For this review, take the finished solid that the model builds, in its own axes (mm). Coordinates: 2 decimals unless noted, no trailing zeros. Write each loop counter-clockwise with the first axis right and the second up, starting at its lowest first coordinate (ties: lowest second). Pieces come first, ordered by that corner, then holes. Notation, with made-up numbers: (-8, 1.5) -> (19, 1.5) arc R28 ccw to (19, 25.5) -> close; hole circle Ø9 at (-39, -37.75). An arc over 180 degrees is marked (long way). Put each result on its own line as item: value. Start each with the question number.
Item 1: Insertion check: P1, Ø1.5, axis at x = 136, y = -2.5, coming from the +Z side. The pin has a flat end and moves straight along its axis. Give the tip position at first contact, or say it passes through.
Item 2: To check wall thickness, follow L1, parallel to Y at x = -21.75, z = 3.15; L2, parallel to X at y = -105, z = 1.25; L3, parallel to Y at x = 175, z = 1. State the ranges of each line that lie inside material, in increasing order.
Item 3: Consider section A-A on y = -95. Give the boundary of the cut face in (x, z), and give its area (3 significant figures).
Item 4: Consider section B-B on z = 5.1. Give the number of separate pieces and of enclosed holes in the cut face, and give its area (3 significant figures).
```python
from build123d import *

# Parameters (mm, degrees)
ESQUISSE1_W             = 280
ESQUISSE1_H             = 200
EXTRUSION1_DEPTH        = 6
ESQUISSE2_W             = 6.5
ESQUISSE2_H             = 140
ENL_V_MAT_EXTRU_1_DEPTH = 2
ESQUISSE3_R             = 1.6
ENL_V_MAT_EXTRU_2_DEPTH = 2
ENL_V_MAT_EXTRU_4_DEPTH = 2
CONG_1_R                = 2.1
ESQUISSE6_W             = 25
ESQUISSE6_H             = 6.5
ESQUISSE6_W_2           = 75.5
ENL_V_MAT_EXTRU_5_DEPTH = 2
ESQUISSE7_R             = 1.6
ENL_V_MAT_EXTRU_6_DEPTH = 2
ESQUISSE4_R             = 1.05
ENL_V_MAT_EXTRU_3_DEPTH = 273.095571445


with BuildPart() as part:
    # Esquisse1 → Extrusion1 (new body)
    with BuildSketch(Plane.XY):
        with Locations((80, -60)):
            Rectangle(ESQUISSE1_W, ESQUISSE1_H)
    extrude(amount=EXTRUSION1_DEPTH)

    # Esquisse2 → Enlèv. mat.-Extru.1 (cut)
    with BuildSketch(Plane.XY.offset(6)):
        with Locations((-21.75, -60)):
            Rectangle(ESQUISSE2_W, ESQUISSE2_H)
        with Locations((54.75, -60)):
            Rectangle(ESQUISSE2_W, ESQUISSE2_H)
        with Locations((131.25, -60)):
            Rectangle(ESQUISSE2_W, ESQUISSE2_H)
    extrude(amount=-ENL_V_MAT_EXTRU_1_DEPTH, mode=Mode.SUBTRACT)

    # Esquisse3 → Enlèv. mat.-Extru.2 (cut)
    with BuildSketch(Plane.XY.offset(6)):
        with Locations((-23.9, 8.9)):
            Circle(ESQUISSE3_R)
        with Locations((-19.6, 8.9)):
            Circle(ESQUISSE3_R)
        with Locations((-23.9, -128.9)):
            Circle(ESQUISSE3_R)
        with Locations((-19.6, -128.9)):
            Circle(ESQUISSE3_R)
        with Locations((52.6, 8.9)):
            Circle(ESQUISSE3_R)
        with Locations((56.9, 8.9)):
            Circle(ESQUISSE3_R)
        with Locations((52.6, -128.9)):
            Circle(ESQUISSE3_R)
        with Locations((56.9, -128.9)):
            Circle(ESQUISSE3_R)
        with Locations((129.1, 8.9)):
            Circle(ESQUISSE3_R)
        with Locations((133.4, 8.9)):
            Circle(ESQUISSE3_R)
        with Locations((129.1, -128.9)):
            Circle(ESQUISSE3_R)
        with Locations((133.4, -128.9)):
            Circle(ESQUISSE3_R)
    extrude(amount=-ENL_V_MAT_EXTRU_2_DEPTH, mode=Mode.SUBTRACT)

    # Esquisse5 → Enlèv. mat.-Extru.4 (cut)
    with BuildSketch(Plane.XY.offset(6)):
        Polygon((86, -53), (86, -81), (100, -81), (100, -53), (107, -53), (93, -39), (79, -53), align=None)
        Polygon((86, -116), (86, -144), (100, -144), (100, -116), (107, -116), (93, -102), (79, -116), align=None)
        Polygon((86, 10), (86, -18), (100, -18), (100, 10), (107, 10), (93, 24), (79, 10), align=None)
        Polygon((9.5, -4), (2.5, -4), (16.5, -18), (30.5, -4), (23.5, -4), (23.5, 24), (9.5, 24), align=None)
        Polygon((9.5, -67), (2.5, -67), (16.5, -81), (30.5, -67), (23.5, -67), (23.5, -39), (9.5, -39), align=None)
        Polygon((9.5, -130), (2.5, -130), (16.5, -144), (30.5, -130), (23.5, -130), (23.5, -102), (9.5, -102), align=None)
    extrude(amount=-ENL_V_MAT_EXTRU_4_DEPTH, mode=Mode.SUBTRACT)

    # Congé1
    cong_1_edges = [part.edges().sort_by_distance(p)[0] for p in [
        (79, -116, 5),
        (93, -102, 5),
        (107, -116, 5),
        (100, -144, 5),
        (86, -144, 5),
        (9.5, 24, 5),
        (23.5, 24, 5),
        (30.5, -4, 5),
        (16.5, -18, 5),
        (2.5, -4, 5),
        (79, -53, 5),
        (93, -39, 5),
        (107, -53, 5),
        (100, -81, 5),
        (86, -81, 5),
        (79, 10, 5),
        (93, 24, 5),
        (107, 10, 5),
        (100, -18, 5),
        (86, -18, 5),
        (9.5, -39, 5),
        (23.5, -39, 5),
        (30.5, -67, 5),
        (16.5, -81, 5),
        (2.5, -67, 5),
        (9.5, -102, 5),
        (23.5, -102, 5),
        (30.5, -130, 5),
        (16.5, -144, 5),
        (2.5, -130, 5),
    ]]
    fillet(cong_1_edges, radius=CONG_1_R)

    # Esquisse6 → Enlèv. mat.-Extru.5 (cut)
    with BuildSketch(Plane.XY.offset(6)):
        with Locations((-37.5, -116.75)):
            Rectangle(ESQUISSE6_W, ESQUISSE6_H)
        with Locations((172.25, -3.25)):
            Rectangle(ESQUISSE6_W_2, ESQUISSE6_H)
    extrude(amount=-ENL_V_MAT_EXTRU_5_DEPTH, mode=Mode.SUBTRACT)

    # Esquisse7 → Enlèv. mat.-Extru.6 (cut)
    with BuildSketch(Plane.XY.offset(6)):
        with Locations((208.9, -1.1)):
            Circle(ESQUISSE7_R)
        with Locations((208.9, -5.4)):
            Circle(ESQUISSE7_R)
        with Locations((-48.9, -114.6)):
            Circle(ESQUISSE7_R)
        with Locations((-48.9, -118.9)):
            Circle(ESQUISSE7_R)
    extrude(amount=-ENL_V_MAT_EXTRU_6_DEPTH, mode=Mode.SUBTRACT)

    # Esquisse4 → Enlèv. mat.-Extru.3 (cut, through all)
    with BuildSketch(Plane.XY.offset(6)):
        with Locations((-21.75, -15)):
            Circle(ESQUISSE4_R)
        with Locations((-21.75, -105)):
            Circle(ESQUISSE4_R)
        with Locations((54.75, -15)):
            Circle(ESQUISSE4_R)
        with Locations((54.75, -105)):
            Circle(ESQUISSE4_R)
        with Locations((131.25, -15)):
            Circle(ESQUISSE4_R)
        with Locations((131.25, -105)):
            Circle(ESQUISSE4_R)
        with Locations((-38, -116.75)):
            Circle(ESQUISSE4_R)
        with Locations((175, -3.25)):
            Circle(ESQUISSE4_R)
    extrude(amount=-ENL_V_MAT_EXTRU_3_DEPTH, mode=Mode.SUBTRACT)


solid = part.part
```
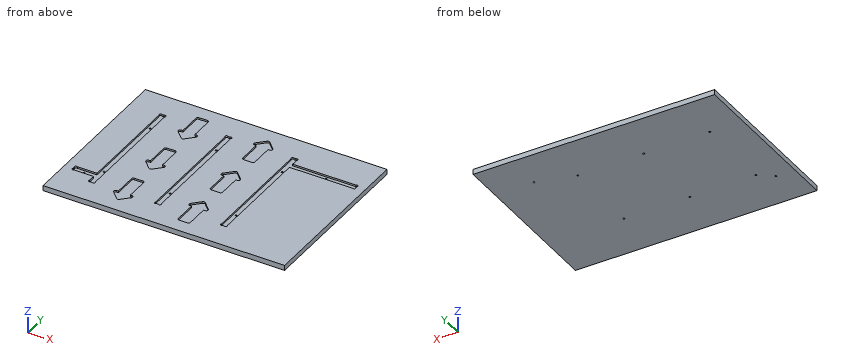
Return value:
1. P1: z = 4
2. L1: -160 to -106.05, -103.95 to -16.05, -13.95 to 40
2. L2: -60 to -22.8, -20.7 to 53.7, 55.8 to 130.2, 132.3 to 220
2. L3: -160 to -4.3, -2.2 to 40
3. outline: (-60, 0) -> (220, 0) -> (220, 6) -> (134.5, 6) -> (134.5, 4) -> (128, 4) -> (128, 6) -> (58, 6) -> (58, 4) -> (51.5, 4) -> (51.5, 6) -> (-18.5, 6) -> (-18.5, 4) -> (-25, 4) -> (-25, 6) -> (-60, 6) -> close
3. area: 1,640 mm^2
4. separate pieces: 1
4. enclosed holes: 9
4. area: 49,100 mm^2
